Source: CAD feature listing. Evaluate the final solid. Frame: model axes, mm. A direction names the side the tool comes from. Give positions to 0.01 mm unless a question says otherwise; leave off trailing zeros. Order: outer loops, then holes, each group sorted by start corner. A loop starts at its lowest first (then second) coordinate and runs counter-clockwise, first axis right, second up. Notation, with made-up numbers: (22.25, 60.25) -> (81.25, 60.25) arc R24 ccw to (81.25, 73.25) -> close; hole circle Ø3 at (83, -36.75). An arc over 180 degrees is marked (long way). Answer in a Markdown table with one row per item.
```python
from build123d import *

# Parameters (mm, degrees)
ESQUISSE1_W                = 10
ESQUISSE1_H                = 19.5
MAIN_DEPTH                 = 5
SKETCH2_W                  = 10
SKETCH2_H                  = 2.9
MAKERBEAMSIDESUPPORT_DEPTH = 10.75
SKETCH3_W                  = 2.9
SKETCH3_H                  = 19.5
MAKERBEAMTOPSUPPORT_DEPTH  = 1
ESQUISSE2_R                = 1.3
SERVOFIXINGHOLES_DEPTH     = 10
ESQUISSE3_R                = 1.3
SIDEHOLES_DEPTH            = 2
SIDEHOLES_DEPTH_BACK       = 11
ESQUISSE4_R                = 1.3
TOPHOLES_DEPTH             = 21.5
SKETCH1_W                  = 3
SKETCH1_H                  = 19.5
BOSS_EXTRUDE1_DEPTH        = 2.5


with BuildPart() as part:
    # Esquisse1 → Main (new body, symmetric)
    with BuildSketch(Plane.XY):
        Rectangle(ESQUISSE1_W, ESQUISSE1_H)
    extrude(amount=MAIN_DEPTH, both=True)

    # Sketch2 → MakerBeamSideSupport (add, symmetric)
    with BuildSketch(Plane(origin=(0, 0, 0), x_dir=(1, 0, 0), z_dir=(0, 1, 0))):
        Rectangle(SKETCH2_W, SKETCH2_H)
    extrude(amount=MAKERBEAMSIDESUPPORT_DEPTH, both=True)

    # Sketch3 → MakerBeamTopSupport (add)
    with BuildSketch(Plane.ZY.offset(5)):
        Rectangle(SKETCH3_W, SKETCH3_H)
    extrude(amount=MAKERBEAMTOPSUPPORT_DEPTH)

    # Esquisse2 → ServoFixingHoles (cut)
    with BuildSketch(Plane(origin=(0, 0, -5), x_dir=(-1, 0, 0), z_dir=(0, 0, -1))):
        with Locations((-0.5, 4.75)):
            Circle(ESQUISSE2_R)
        with Locations((-0.5, -4.75)):
            Circle(ESQUISSE2_R)
    extrude(amount=-SERVOFIXINGHOLES_DEPTH, mode=Mode.SUBTRACT)

    # Esquisse3 → SideHoles (cut, two sides)
    with BuildSketch(Plane.ZY.offset(5)) as sideholes_sk:
        Circle(ESQUISSE3_R)
    extrude(amount=SIDEHOLES_DEPTH, mode=Mode.SUBTRACT)
    extrude(sideholes_sk.sketch, amount=-SIDEHOLES_DEPTH_BACK, mode=Mode.SUBTRACT)

    # Esquisse4 → TopHoles (cut, through all)
    with BuildSketch(Plane.XZ.offset(9.75)):
        Circle(ESQUISSE4_R)
    extrude(amount=-TOPHOLES_DEPTH, mode=Mode.SUBTRACT)

    # Sketch1 → Boss-Extrude1 (add)
    with BuildSketch(Plane(origin=(0, 0, -5), x_dir=(-1, 0, 0), z_dir=(0, 0, -1))):
        with Locations((3.5, 0)):
            Rectangle(SKETCH1_W, SKETCH1_H)
    extrude(amount=BOSS_EXTRUDE1_DEPTH)


solid = part.part
```
(1) Section query D-D (z = -3.75). Return the cut outline in (x, y).
A:
| item | result |
|---|---|
| outline | (-5, -9.75) -> (5, -9.75) -> (5, 9.75) -> (-5, 9.75) -> close; hole circle Ø2.6 at (0.5, -4.75); hole circle Ø2.6 at (0.5, 4.75) |
(2) Pull-direction query (Z, two-part tool) for faces 5 (the cylindrical face through (-3.71, 0.06, -1.3)), 6 (the flat face through (0, -10.75, 0)), 7 (the cylindrical face through (-1.3, 6.49, 0.06)), 8 (the flat face through (-5.5, -0.1, -1.45)); classes: +Z half, -Z half, draft (parallel to the pull), parting line (faces both ways), or undercut.
A:
| item | result |
|---|---|
| face 5 | undercut |
| face 6 | draft |
| face 7 | undercut |
| face 8 | -Z half |
(3) Section query C-C (z = 0). Return the cut outline in (x, y), plus the area to 3 significant figures.
A:
| item | result |
|---|---|
| outline | (-6, -9.75) -> (-5, -9.75) -> (-5, -10.75) -> (5, -10.75) -> (5, -1.3) -> (1.3, -1.3) -> (1.3, -3.73) arc R1.3 cw to (1.3, -5.77) -> (1.3, -9.75) -> (-1.3, -9.75) -> (-1.3, -1.3) -> (-6, -1.3) -> close; (-6, 1.3) -> (-1.3, 1.3) -> (-1.3, 10.75) -> (-5, 10.75) -> (-5, 9.75) -> (-6, 9.75) -> close; (1.3, 1.3) -> (5, 1.3) -> (5, 10.75) -> (1.3, 10.75) -> (1.3, 5.77) arc R1.3 cw to (1.3, 3.73) -> close |
| area | 158 mm^2 |
(4) Section query A-A (y = -8.25). Return the cut outline in (x, z), plus the area to 3 significant figures.
A:
| item | result |
|---|---|
| outline | (-6, -1.45) -> (-5, -1.45) -> (-5, -7.5) -> (-2, -7.5) -> (-2, -5) -> (5, -5) -> (5, 5) -> (-5, 5) -> (-5, 1.45) -> (-6, 1.45) -> close; hole circle Ø2.6 at (0, 0) |
| area | 105 mm^2 |
(5) Access query for faces 1 (the flat face through (-1, -9.75, -4)), 2 (the flat face through (-5.5, -0.1, 1.45)), 3 (the flat face through (-5, -10, 0)), 4 (the flat face through (-1, 9.75, -4)). Directions: +Z, -Z, +X, -X, +Y, -Y. A direction counts if a zero-diameter tool reaches every point of the face in a straight line with its end or side. Return the directions, or none.
A:
| item | result |
|---|---|
| face 1 | -Z, +X, -X, -Y |
| face 2 | +Z, -X, +Y, -Y |
| face 3 | +Z, -Z, -X, -Y |
| face 4 | -Z, +X, -X, +Y |
(6) First-contact query: pin 1 Ø5.5 at (x, y) = (2, -4.5) entering from -Z; pin 2 Ø1.2 at (y, z) = (-1.5, -6.5) entering from +X; pin 3 Ø4 at (y, z) = (-1, 3.5) entering from -X; pin 4 Ø2.5 at (y, z) = (0, 0) entering from -X. Flat tips, straight axial feed; report the tip coordinate or a pass-through.
A:
| item | result |
|---|---|
| pin 1 | stops at z = -5 |
| pin 2 | stops at x = -2 |
| pin 3 | stops at x = -5 |
| pin 4 | passes through |
(7) Ray query, probe 1 along Y at (x, z) = (2.2, 0); probe 2 along Z at (x, y) = (-1.15, 0); probe 3 along X at (y, z) = (-3.25, -1.5). Return the intervals inside material, ascending.
A:
| item | result |
|---|---|
| probe 1 | y = -10.75 to -1.3, 1.3 to 10.75 |
| probe 2 | z = -5 to -1.3, 1.3 to 5 |
| probe 3 | x = -5 to 5 |
(8) Section query B-B (x = -4.5). Return the cut outline in (y, z).
A:
| item | result |
|---|---|
| outline | (-10.75, -1.45) -> (-9.75, -1.45) -> (-9.75, -7.5) -> (9.75, -7.5) -> (9.75, -1.45) -> (10.75, -1.45) -> (10.75, 1.45) -> (9.75, 1.45) -> (9.75, 5) -> (-9.75, 5) -> (-9.75, 1.45) -> (-10.75, 1.45) -> close; hole circle Ø2.6 at (0, 0) |
